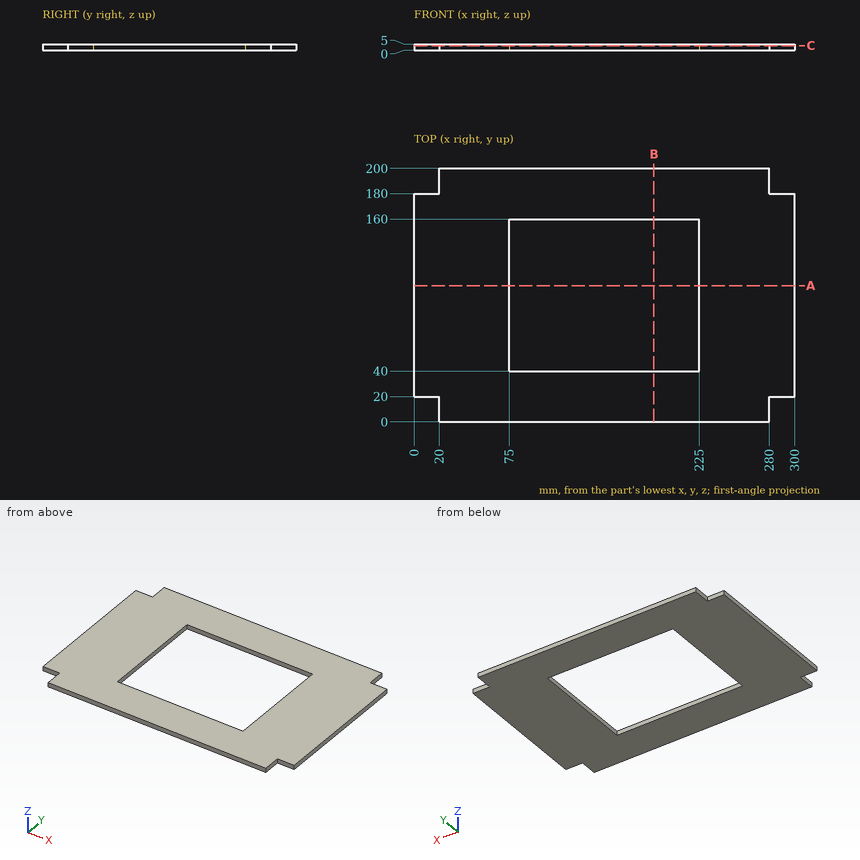
Design review of the part shown in the three views and the two pictorial views. Dimensions are in mm from the part's minimum x, y and z. Give positions to 0.01 mm unless a question says otherwise; leave off trailing zeros. Write each loop counter-clockwise with the first axis right and the second up, starting at its lowest first coordinate (ties: lowest second). Pieces come first, ordered by that corner, then holes. Notation, with made-up numbers: M 4,-38 L 14,-38 A22 ccw 14,-5 Z; hole C 47.25,35.25 d2. An arc over 180 degrees is marked long. One line per item, written item: value.
1) For P1, Ø2.5, axis at y = 12, z = 3, coming from the -X side; P2, Ø1.5, axis at x = 7, z = 3, coming from the -Y side; P3, Ø2.5, axis at y = 190.5, z = 3, coming from the +X side, all flat-tipped, find the tip position at first contact; note any pin that passes through.
Results are:
P1: stops at x = 20
P2: stops at y = 20
P3: stops at x = 280
2) Take a section at B-B, the plane x = 189. Write out the cut boundary in (y, z), then the cut area to 3 significant figures.
Results are:
outline: M 0,0 L 40,0 L 40,5 L 0,5 Z; M 160,0 L 200,0 L 200,5 L 160,5 Z
area: 400 mm²
3) Take a section at A-A, the plane y = 107.5. Write out the cut boundary in (x, z).
Results are:
outline: M 0,0 L 75,0 L 75,5 L 0,5 Z; M 225,0 L 300,0 L 300,5 L 225,5 Z
4) For line 1 (X direction, y = 71, z = 1.25); line 2 (Y direction, x = 95.5, z = 3.55); line 3 (X direction, y = 182, z = 1.2), list the stretches that pass through material, from the lowest coordinate up. Write a range as from..to.
Results are:
line 1: x = 0..75, 225..300
line 2: y = 0..40, 160..200
line 3: x = 20..280
5) Take a section at C-C, the plane z = 3.65. Write out the cut boundary in (x, y), then the cut area to 3 significant figures.
Results are:
outline: M 0,20 L 20,20 L 20,0 L 280,0 L 280,20 L 300,20 L 300,180 L 280,180 L 280,200 L 20,200 L 20,180 L 0,180 Z; hole M 75,40 L 225,40 L 225,160 L 75,160 Z
area: 40,400 mm²
